For this review, take the finished solid that the model builds, in its own axes (mm). Face numbers are marked on the shaded views. Give positions to 0.01 mm unless a question says otherwise; leave off trailing zeros. Loops run counter-clockwise (first coordinate to the right, second up) from the corner with the lowest first, then second, coordinate; pieces in that order, holes last.
```python
from build123d import *

# Parameters (mm, degrees)
SKETCH_W          = 81
SKETCH_H          = 81
PAD_DEPTH         = 20
POCKET_DEPTH      = 40.501
POCKET_DEPTH_BACK = -40.501
SKETCH001_W       = 83
SKETCH001_H       = 83
PAD001_DEPTH      = 21
FILLET_R          = 1


with BuildPart() as body:
    # Sketch → Pad (new body)
    with BuildSketch(Plane.XY):
        Rectangle(SKETCH_W, SKETCH_H)
    extrude(amount=PAD_DEPTH)

    # Sketch002 → Pocket (cut, two sides)
    with BuildSketch(Plane.YZ) as pocket_sk:
        with BuildLine():
            ThreePointArc((40.5, 4.5), (40, 4), (40.5, 3.5))
            Line((40.5, 4.5), (40.5, 3.5))
        make_face()
        with BuildLine():
            ThreePointArc((-40.5, 3.5), (-40, 4), (-40.5, 4.5))
            Line((-40.5, 3.5), (-40.5, 4.5))
        make_face()
    extrude(amount=-POCKET_DEPTH, mode=Mode.SUBTRACT)
    extrude(pocket_sk.sketch, amount=-POCKET_DEPTH_BACK, mode=Mode.SUBTRACT)


with BuildPart() as body001:
    # Sketch001 → Pad001 (new body)
    with BuildSketch(Plane.XY):
        Rectangle(SKETCH001_W, SKETCH001_H)
    extrude(amount=PAD001_DEPTH)

    # Fillet
    fillet_edges = [body001.edges().sort_by_distance(p)[0] for p in [
        (-41.5, -41.5, 10.5),
        (0, -41.5, 21),
        (41.5, -41.5, 10.5),
        (41.5, 0, 21),
        (41.5, 41.5, 10.5),
        (0, 41.5, 21),
        (-41.5, 0, 21),
        (-41.5, 41.5, 10.5),
    ]]
    fillet(fillet_edges, radius=FILLET_R)

    # Boolean: cut Body
    add(body.part, mode=Mode.SUBTRACT)


solid = body001.part
```
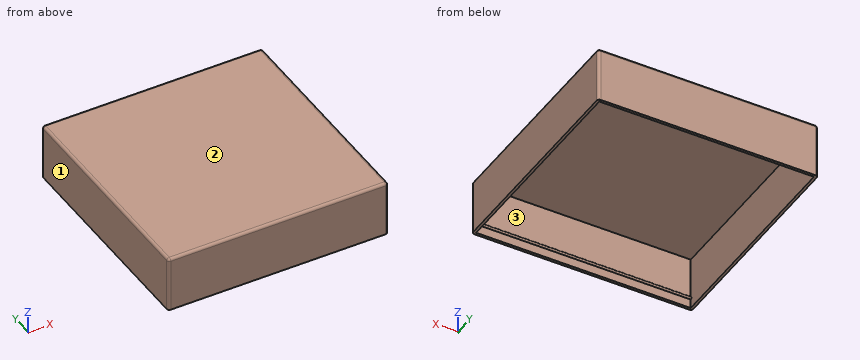
Item 1: Take a section at C-C on y = 28.5. Give the boundary of the cut face in (x, z), and give its area (3 significant figures).
Answer:
outline: (-41.5, 0) - (-40.5, 0) - (-40.5, 20) - (40.5, 20) - (40.5, 0) - (41.5, 0) - (41.5, 20) arc R1 ccw to (40.5, 21) - (-40.5, 21) arc R1 ccw to (-41.5, 20) - close
area: 123 mm2
Item 2: Take a section at B-B on x = -29.5. Give the boundary of the cut face in (y, z).
Answer:
outline: (-41.5, 0) - (-40.5, 0) - (-40.5, 3.5) arc R0.5 ccw to (-40.5, 4.5) - (-40.5, 20) - (40.5, 20) - (40.5, 4.5) arc R0.5 ccw to (40.5, 3.5) - (40.5, 0) - (41.5, 0) - (41.5, 20) arc R1 ccw to (40.5, 21) - (-40.5, 21) arc R1 ccw to (-41.5, 20) - close
Item 3: For L1, parallel to X at y = -16.5, z = 7.25; L2, parallel to Z at x = 22.5, y = 17.5, list the stretches that pass through material, from the lowest coordinate up.
Answer:
L1: x = -41.5 to -40.5, 40.5 to 41.5
L2: z = 20 to 21
Item 4: The part is to be moulded in two halves that separate along Z. For the marked faces 1, 2 and 3, say which applies: released by +Z, released by -Z, zero draft, split by the parting line, or undercut.
Answer:
face 1: zero draft
face 2: released by +Z
face 3: undercut
Item 5: Take a section at A-A on z = 1.5. Give the boundary of the cut face in (x, y).
Answer:
outline: (-41.5, -40.5) arc R1 ccw to (-40.5, -41.5) - (40.5, -41.5) arc R1 ccw to (41.5, -40.5) - (41.5, 40.5) arc R1 ccw to (40.5, 41.5) - (-40.5, 41.5) arc R1 ccw to (-41.5, 40.5) - close; hole (-40.5, -40.5) - (40.5, -40.5) - (40.5, 40.5) - (-40.5, 40.5) - close
Item 6: Clearance check with a flat-ended pin moving along its axis: pin 1 Ø6 at (x, y) = (6.5, -8) entering from -Z. State where the tip first meets the part, or that it passes through.
Answer:
pin 1: stops at z = 20
